Input: part model. Units: mm. Frame: model coordinates. Give positions to 0.01 mm unless a question says otherwise; leave off trailing zeros. Write each loop counter-clockwise with the first axis right and the second up, starting at its lowest first coordinate (ties: lowest second). Pieces come first, ordered by that corner, then holes. Notation, with made-up numbers: (-6.75, 66.5) - (42.25, 66.5) arc R33 ccw to (42.25, 104.5) - close; hole circle Ø2 at (65.25, 51.25). An arc over 180 degrees is marked (long way). Answer as a JSON object with one key per item and string values. Group by question number.
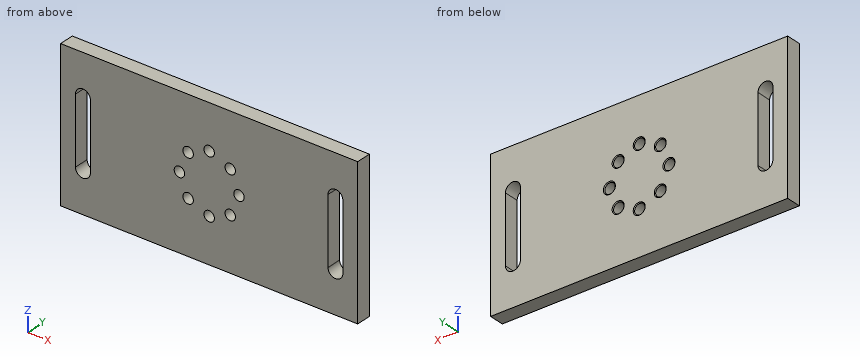
from build123d import *

# Parameters (mm, degrees)
SKETCH2_W                       = 200
SKETCH2_H                       = 100
BOSS_EXTRUDE2_DEPTH             = 10
M8X1_0_TAPPED_HOLE1_D           = 7
M8X1_0_TAPPED_HOLE1_CSINK_D     = 8.05
M8X1_0_TAPPED_HOLE1_CSINK_ANGLE = 90
CIRPATTERN1_COUNT               = 8
CUT_EXTRUDE1_DEPTH              = 224.830292856


with BuildPart() as part:
    # Sketch2 → Boss-Extrude2 (new body)
    with BuildSketch(Plane(origin=(0, 0, 0), x_dir=(1, 0, 0), z_dir=(0, 1, 0))):
        with Locations((100, 50)):
            Rectangle(SKETCH2_W, SKETCH2_H)
    extrude(amount=BOSS_EXTRUDE2_DEPTH)

    # M8x1.0 Tapped Hole1 (through all)
    with Locations(Plane(origin=(0, 10, 0), x_dir=(1, 0, 0), z_dir=(0, 1, 0))):
        with Locations((100, 70)):
            m8x1_0_tapped_hole1 = CounterSinkHole(M8X1_0_TAPPED_HOLE1_D / 2, M8X1_0_TAPPED_HOLE1_CSINK_D / 2, counter_sink_angle=M8X1_0_TAPPED_HOLE1_CSINK_ANGLE)

    # CirPattern1: M8x1.0 Tapped Hole1 ×8 about axis
    cirpattern1_axis = Axis((100, 0, -49.948974386), (0, 1, 0))
    for i in range(1, CIRPATTERN1_COUNT):
        add(m8x1_0_tapped_hole1.rotate(cirpattern1_axis, i * 360 / CIRPATTERN1_COUNT), mode=Mode.SUBTRACT)

    # Sketch6 → Cut-Extrude1 (cut, through all)
    with BuildSketch(Plane(origin=(0, 10, 0), x_dir=(1, 0, 0), z_dir=(0, 1, 0))):
        with BuildLine():
            Line((20, 72.5), (20, 27.5))
            ThreePointArc((20, 27.5), (15, 22.5), (10, 27.5))
            Line((10, 27.5), (10, 72.5))
            ThreePointArc((10, 72.5), (15, 77.5), (20, 72.5))
        make_face()
        with BuildLine():
            Line((180, 72.5), (180, 27.5))
            ThreePointArc((180, 27.5), (185, 22.5), (190, 27.5))
            Line((190, 27.5), (190, 72.5))
            ThreePointArc((190, 72.5), (185, 77.5), (180, 72.5))
        make_face()
    extrude(amount=-CUT_EXTRUDE1_DEPTH, mode=Mode.SUBTRACT)


solid = part.part
1) Cut plane B-B on x = 185. Return the cut outline in (y, z), and give its area (3 significant figures).
2) Line query: line 1 along Z through (x, y) = (100, 3.25); line 2 along Z through (x, y) = (79.5, 5); line 3 along X through (y, z) = (1, -56). Output: solid intervals per line, ascending. Write a range as from..to.
3) Cut plane A-A on x = 100. Return the cut outline in (y, z) (3 decimals), and give its area (3 significant figures).
4) Cut plane C-C on z = -70. Return the cut outline in (x, y) (3 decimals), and give its area (3 significant figures).
5) Cut plane D-D on y = 7.5. Count the separate pieces of the cut face and the enclosed holes in it, and give its area (3 significant figures).
Filled in:
{
 "1": {"outline": "(0, -100) - (10, -100) - (10, -77.5) - (0, -77.5) - close; (0, -22.5) - (10, -22.5) - (10, 0) - (0, 0) - close", "area": "450 mm²"},
 "2": {"line 1": "z = -100..-73.5, -66.5..-33.4, -26.4..0", "line 2": "z = -100..-53.42, -46.48..0", "line 3": "x = 0..10, 20..180, 190..200"},
 "3": {"outline": "(0, -100) - (10, -100) - (10, -74.025) - (9.475, -73.5) - (0, -73.5) - close; (0, -66.5) - (9.475, -66.5) - (10, -65.975) - (10, -33.923) - (9.475, -33.398) - (0, -33.398) - close; (0, -26.398) - (9.475, -26.398) - (10, -25.873) - (10, 0) - (0, 0) - close", "area": "859 mm²"},
 "4": {"outline": "(0, 0) - (10, 0) - (10, 10) - (0, 10) - close; (20, 0) - (96.5, 0) - (96.5, 9.475) - (95.975, 10) - (20, 10) - close; (103.5, 0) - (180, 0) - (180, 10) - (104.025, 10) - (103.5, 9.475) - close; (190, 0) - (200, 0) - (200, 10) - (190, 10) - close", "area": "1,730 mm²"},
 "5": {"separate pieces": "1", "enclosed holes": "10", "area": "18,600 mm²"}
}
